```python
from build123d import *

# Parameters (mm, degrees)
SKETCH1_W           = 80
SKETCH1_H           = 48
SKETCH1_R           = 7
SKETCH1_R_2         = 2.05
BOSS_EXTRUDE1_DEPTH = 3.175
FILLET1_R           = 8


with BuildPart() as part:
    # Sketch1 → Boss-Extrude1 (new body)
    with BuildSketch(Plane.XY):
        Rectangle(SKETCH1_W, SKETCH1_H)
        with Locations((-24, 0)):
            Circle(SKETCH1_R, mode=Mode.SUBTRACT)
        with Locations((-32, 16)):
            Circle(SKETCH1_R_2, mode=Mode.SUBTRACT)
        with Locations((-16, 16)):
            Circle(SKETCH1_R_2, mode=Mode.SUBTRACT)
        with Locations((0, 16)):
            Circle(SKETCH1_R_2, mode=Mode.SUBTRACT)
        with Locations((16, 16)):
            Circle(SKETCH1_R_2, mode=Mode.SUBTRACT)
        with Locations((32, 16)):
            Circle(SKETCH1_R_2, mode=Mode.SUBTRACT)
        with Locations((-16, 8)):
            Circle(SKETCH1_R_2, mode=Mode.SUBTRACT)
        with Locations((0, 8)):
            Circle(SKETCH1_R_2, mode=Mode.SUBTRACT)
        with Locations((16, 8)):
            Circle(SKETCH1_R_2, mode=Mode.SUBTRACT)
        with Locations((32, 8)):
            Circle(SKETCH1_R_2, mode=Mode.SUBTRACT)
        Circle(SKETCH1_R_2, mode=Mode.SUBTRACT)
        with Locations((16, 0)):
            Circle(SKETCH1_R_2, mode=Mode.SUBTRACT)
        with Locations((32, 0)):
            Circle(SKETCH1_R_2, mode=Mode.SUBTRACT)
        with Locations((-16, -8)):
            Circle(SKETCH1_R_2, mode=Mode.SUBTRACT)
        with Locations((0, -8)):
            Circle(SKETCH1_R_2, mode=Mode.SUBTRACT)
        with Locations((16, -8)):
            Circle(SKETCH1_R_2, mode=Mode.SUBTRACT)
        with Locations((32, -8)):
            Circle(SKETCH1_R_2, mode=Mode.SUBTRACT)
        with Locations((-16, -16)):
            Circle(SKETCH1_R_2, mode=Mode.SUBTRACT)
        with Locations((0, -16)):
            Circle(SKETCH1_R_2, mode=Mode.SUBTRACT)
        with Locations((16, -16)):
            Circle(SKETCH1_R_2, mode=Mode.SUBTRACT)
        with Locations((32, -16)):
            Circle(SKETCH1_R_2, mode=Mode.SUBTRACT)
        with Locations((-32, 8)):
            Circle(SKETCH1_R_2, mode=Mode.SUBTRACT)
        with Locations((-32, -8)):
            Circle(SKETCH1_R_2, mode=Mode.SUBTRACT)
        with Locations((-32, -16)):
            Circle(SKETCH1_R_2, mode=Mode.SUBTRACT)
    extrude(amount=BOSS_EXTRUDE1_DEPTH)

    # Fillet1
    fillet1_edges = [part.edges().sort_by_distance(p)[0] for p in [
        (-40, 24, 1.5875),
        (40, 24, 1.5875),
        (40, -24, 1.5875),
        (-40, -24, 1.5875),
    ]]
    fillet(fillet1_edges, radius=FILLET1_R)


solid = part.part
```
Model file for the job. Use its own axes, mm. Coordinates: 2 decimals unless noted, no trailing zeros. Loops run counter-clockwise (first coordinate to the right, second up) from the corner with the lowest first, then second, coordinate; pieces in that order, holes last. Notation, with made-up numbers: (68.25, 19.25) - (89.25, 19.25) arc R23 ccw to (89.25, 56.25) - close; hole circle Ø5 at (8, 85.5). An arc over 180 degrees is marked (long way). Answer as a JSON object with one key per item and string values. Group by question number.
(1) Cut at B-B (x = -16). Give the cut face in (y, z) (3 decimals), then the cut area to 3 significant figures.
(2) Cut at C-C (x = -24). Give the cut face in (y, z) (3 decimals).
(3) Probe line 1 along Y through (x, z) = (-32, 1.2); line 2 along Y through (x, z) = (32, 2.3); line 3 along X through (y, z) = (-15, 1.1). List the from-to ranges inside material, lowest first.
(4) Cut at D-D (z = 1.4). State how many separate pieces and enclosed holes the cut face has, then the cut area to 3 significant figures.
(5) Two-plate mould, pull along Y, no slides. Class faces 1 (the face through (0, 24, 2)), 2 (the face through (40, 0, 2)), 3 (the face through (-17.5, 17.4, 1.6)): released by +Y, released by -Y, zero draft, split by the parting line, or undercut.
(6) Cut at A-A (y = 0). Give the cut face in (x, z) (3 decimals).
Geometry says:
{
 "1": {"outline": "(-24, 0) - (-18.05, 0) - (-18.05, 3.175) - (-24, 3.175) - close; (-13.95, 0) - (-10.05, 0) - (-10.05, 3.175) - (-13.95, 3.175) - close; (-5.95, 0) - (5.95, 0) - (5.95, 3.175) - (-5.95, 3.175) - close; (10.05, 0) - (13.95, 0) - (13.95, 3.175) - (10.05, 3.175) - close; (18.05, 0) - (24, 0) - (24, 3.175) - (18.05, 3.175) - close", "area": "100 mm^2"},
 "2": {"outline": "(-24, 0) - (-7, 0) - (-7, 3.175) - (-24, 3.175) - close; (7, 0) - (24, 0) - (24, 3.175) - (7, 3.175) - close"},
 "3": {"line 1": "y = -24 to -18.05, -13.95 to -10.05, -5.95 to 5.95, 10.05 to 13.95, 18.05 to 24", "line 2": "y = -24 to -18.05, -13.95 to -10.05, -5.95 to -2.05, 2.05 to 5.95, 10.05 to 13.95, 18.05 to 24", "line 3": "x = -40 to -33.79, -30.21 to -17.79, -14.21 to -1.79, 1.79 to 14.21, 17.79 to 30.21, 33.79 to 40"},
 "4": {"separate pieces": "1", "enclosed holes": "24", "area": "3,330 mm^2"},
 "5": {"face 1": "released by +Y", "face 2": "zero draft", "face 3": "undercut"},
 "6": {"outline": "(-40, 0) - (-31, 0) - (-31, 3.175) - (-40, 3.175) - close; (-17, 0) - (-2.05, 0) - (-2.05, 3.175) - (-17, 3.175) - close; (2.05, 0) - (13.95, 0) - (13.95, 3.175) - (2.05, 3.175) - close; (18.05, 0) - (29.95, 0) - (29.95, 3.175) - (18.05, 3.175) - close; (34.05, 0) - (40, 0) - (40, 3.175) - (34.05, 3.175) - close"}
}
